from build123d import *

# Parameters (mm, degrees)
SKETCH1_W             = 50.8
SKETCH1_H             = 215.9
BOSS_EXTRUDE1_DEPTH   = 6.35
SKETCH2_R             = 9.398
CUT_EXTRUDE1_DEPTH    = 6.35
LPATTERN1_COUNT       = 3
LPATTERN1_PITCH       = 38.1
LPATTERN1_COL_COUNT   = 3
LPATTERN1_COL_PITCH   = 38.1
F_6_CLEARANCE_HOLE1_D = 3.6576
FILLET1_R             = 6.35


with BuildPart() as part:
    # Sketch1 → Boss-Extrude1 (new body)
    with BuildSketch(Plane.XY):
        Rectangle(SKETCH1_W, SKETCH1_H)
    extrude(amount=BOSS_EXTRUDE1_DEPTH)

    # Sketch2 → Cut-Extrude1 (cut)
    with BuildSketch(Plane.XY.offset(6.35)):
        Circle(SKETCH2_R)
    cut_extrude1 = extrude(amount=-CUT_EXTRUDE1_DEPTH, mode=Mode.SUBTRACT)

    # LPattern1: Cut-Extrude1 ×3
    with Locations(*[(0, -i * LPATTERN1_PITCH, 0) for i in range(1, LPATTERN1_COUNT)]):
        add(cut_extrude1, mode=Mode.SUBTRACT)

    # LPattern1 col: Cut-Extrude1 ×3
    with Locations(*[(0, i * LPATTERN1_COL_PITCH, 0) for i in range(1, LPATTERN1_COL_COUNT)]):
        add(cut_extrude1, mode=Mode.SUBTRACT)

    # #6 Clearance Hole1 (through all)
    with Locations(Plane.XY.offset(6.35)):
        with Locations((19.05, -101.6), (0, 0), (19.05, 101.6), (-19.05, -101.6), (-19.05, 101.6)):
            Hole(F_6_CLEARANCE_HOLE1_D / 2)

    # Fillet1
    fillet1_edges = [part.edges().sort_by_distance(p)[0] for p in [
        (25.4, -107.95, 3.175),
        (-25.4, -107.95, 3.175),
        (-25.4, 107.95, 3.175),
        (25.4, 107.95, 3.175),
    ]]
    fillet(fillet1_edges, radius=FILLET1_R)


solid = part.part
Geometry: final body of the model. Coordinates: model frame, mm. Give positions to 0.01 mm unless a question says otherwise; leave off trailing zeros. Order: outer loops, then holes, each group sorted by start corner. A loop starts at its lowest first (then second) coordinate and runs counter-clockwise, first axis right, second up. Notation, with made-up numbers: (5, 51) -> (43, 51) arc R6 cw to (43, 61) -> close; hole circle Ø10 at (76, 14). An arc over 180 degrees is marked (long way). Answer as a JSON object with one key per item and string values.
Q1. Section C-C (y = 0). Output: boundary loops of the cut face in (x, z).
Entries:
{"outline": "(-25.4, 0) -> (-9.4, 0) -> (-9.4, 6.35) -> (-25.4, 6.35) -> close; (9.4, 0) -> (25.4, 0) -> (25.4, 6.35) -> (9.4, 6.35) -> close"}
Q2. Draft query along X for faces 1 (the flat face through (11, 2, 0)), 2 (the cylindrical face through (4.337, -46.438, 3.219)), 3 (the cylindrical face through (-23.59, 106.04, 3.22)), 4 (the cylindrical face through (23.49, 106.14, 3.22)). Return one class per face: released by +X, released by -X, zero draft, split by the parting line, or undercut.
Entries:
{"face 1": "zero draft", "face 2": "undercut", "face 3": "released by -X", "face 4": "released by +X"}
Q3. Material intervals for probe 1 along Y at (x, z) = (0, 3.5); probe 2 along Y at (x, z) = (19.05, 4); probe 3 along Y at (x, z) = (6, 5), sorted ascending.
Entries:
{"probe 1": "y = -107.95 to -85.6, -66.8 to -47.5, -28.7 to -9.4, 9.4 to 28.7, 47.5 to 66.8, 85.6 to 107.95", "probe 2": "y = -107.95 to -103.43, -99.77 to 99.77, 103.43 to 107.95", "probe 3": "y = -107.95 to -83.43, -68.97 to -45.33, -30.87 to -7.23, 7.23 to 30.87, 45.33 to 68.97, 83.43 to 107.95"}
Q4. Section B-B (z = 1.75). State how many separate pieces and enclosed holes the cut face has, plus the area to 3 significant figures.
Entries:
{"separate pieces": "1", "enclosed holes": "9", "area": "9,500 mm^2"}
Q5. Section D-D (y = -45). Output: boundary loops of the cut face in (x, z).
Entries:
{"outline": "(-25.4, 0) -> (-6.38, 0) -> (-6.38, 6.35) -> (-25.4, 6.35) -> close; (6.38, 0) -> (25.4, 0) -> (25.4, 6.35) -> (6.38, 6.35) -> close"}
Q6. Section A-A (x = 0). Output: boundary loops of the cut face in (y, z), plus the area to 3 significant figures.
Entries:
{"outline": "(-107.95, 0) -> (-85.6, 0) -> (-85.6, 6.35) -> (-107.95, 6.35) -> close; (-66.8, 0) -> (-47.5, 0) -> (-47.5, 6.35) -> (-66.8, 6.35) -> close; (-28.7, 0) -> (-9.4, 0) -> (-9.4, 6.35) -> (-28.7, 6.35) -> close; (9.4, 0) -> (28.7, 0) -> (28.7, 6.35) -> (9.4, 6.35) -> close; (47.5, 0) -> (66.8, 0) -> (66.8, 6.35) -> (47.5, 6.35) -> close; (85.6, 0) -> (107.95, 0) -> (107.95, 6.35) -> (85.6, 6.35) -> close", "area": "774 mm^2"}
